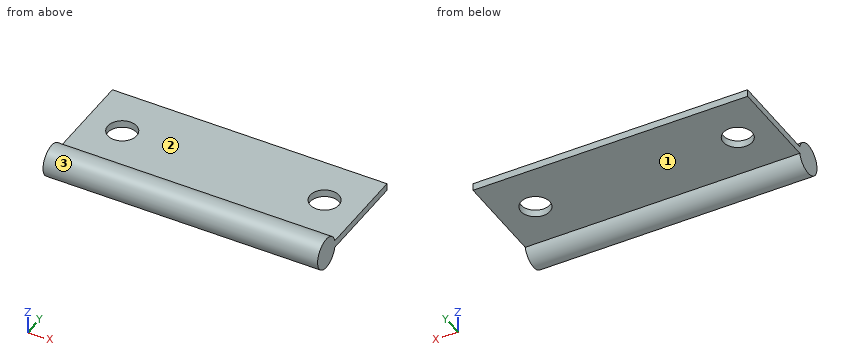
```python
from build123d import *

# Parameters (mm, degrees)
SKETCH_1_W          = 38
SKETCH_1_H          = 30
SKETCH_1_R          = 2
EXTRUDE_1_DEPTH     = 1
SKETCH_2_W          = 38
SKETCH_2_H          = 15
CUT_EXTRUDE_1_DEPTH = 1
SKETCH_4_R          = 2.15
EXTRUDE_2_DEPTH     = 38


with BuildPart() as part:
    # 草图1 → 凸台-拉伸1 (new body)
    with BuildSketch(Plane.XY):
        with Locations((-26.818488663, 4.019613274)):
            Rectangle(SKETCH_1_W, SKETCH_1_H)
        with Locations((-40.818488663, 12.519613274)):
            Circle(SKETCH_1_R, mode=Mode.SUBTRACT)
        with Locations((-12.818488663, 12.519613274)):
            Circle(SKETCH_1_R, mode=Mode.SUBTRACT)
        with Locations((-40.818488663, -4.480386726)):
            Circle(SKETCH_1_R, mode=Mode.SUBTRACT)
        with Locations((-12.818488663, -4.480386726)):
            Circle(SKETCH_1_R, mode=Mode.SUBTRACT)
    extrude(amount=EXTRUDE_1_DEPTH)

    # 草图2 → 切除-拉伸1 (cut)
    with BuildSketch(Plane.XY.offset(1)):
        with Locations((-26.818488663, -3.480386726)):
            Rectangle(SKETCH_2_W, SKETCH_2_H)
    extrude(amount=-CUT_EXTRUDE_1_DEPTH, mode=Mode.SUBTRACT)

    # 草图4 → 凸台-拉伸2 (add)
    with BuildSketch(Plane.ZY.offset(45.818488663)):
        with Locations((0.5, 4.019613274)):
            Circle(SKETCH_4_R)
    extrude(amount=-EXTRUDE_2_DEPTH)


solid = part.part
```
Here's how the part is built. I have some questions about the finished solid (model axes, mm). Face numbers are marked on the shaded views. A direction names the side the tool comes from. Coordinates: 2 decimals unless noted, no trailing zeros. Write each loop counter-clockwise with the first axis right and the second up, starting at its lowest first coordinate (ties: lowest second). Pieces come first, ordered by that corner, then holes. Notation, with made-up numbers: (-6.75, 16) - (14.25, 16) arc R27 cw to (14.25, 46) - close; hole circle Ø1 at (39.5, 3). An arc over 180 degrees is marked (long way). One line per item, written item: value.
1) Suppose I cut it at C-C on z = 0.5. Write out the boundary of the cut face in (x, y).
Model answer:
outline: (-45.82, 1.87) - (-7.82, 1.87) - (-7.82, 19.02) - (-45.82, 19.02) - close; hole circle Ø4 at (-40.82, 12.52); hole circle Ø4 at (-12.82, 12.52)
2) I'm going to push flat-ended pins straight in: P1, Ø4.5, axis at x = -40.82, y = 12.52, coming from the +Z side; P2, Ø4, axis at x = -29, y = 14, coming from the -Z side; P3, Ø1, axis at x = -31, z = -0.5, coming from the -Y side; P4, Ø3, axis at x = -12.82, y = 12.52, coming from the -Z side. Where does each tip first touch, or does it pass through?
Model answer:
P1: stops at z = 1
P2: stops at z = 0
P3: stops at y = 1.93
P4: passes through
3) Suppose I cut it at A-A on x = -13.5. Write out the boundary of the cut face in (y, z).
Model answer:
outline: (6.11, 0) - (10.64, 0) - (10.64, 1) - (6.11, 1) arc R2.15 ccw (long way) to start; (14.4, 0) - (19.02, 0) - (19.02, 1) - (14.4, 1) - close
4) Suppose I cut it at D-D on y = 13.75. Write out the boundary of the cut face in (x, z).
Model answer:
outline: (-45.82, 0) - (-42.4, 0) - (-42.4, 1) - (-45.82, 1) - close; (-39.24, 0) - (-14.4, 0) - (-14.4, 1) - (-39.24, 1) - close; (-11.24, 0) - (-7.82, 0) - (-7.82, 1) - (-11.24, 1) - close
5) On a 3-axis mill with a long thin cutter (end or side, diameter ignored), from which of +Z, -Z, +X, -X, +Y, -Y can I reach the whole of each face in a straight line? I mean the marked faces 1, 2 and 3. Say none if no direction works.
Model answer:
face 1: -Z, +X, -X, +Y
face 2: +Z, +X, -X, +Y
face 3: +X, -X
6) I need wall thicknesses on line 1 along X through (y, z) = (12.5, 0.6); line 2 along Z through (x, y) = (-41.5, 7); line 3 along Y through (x, z) = (-11.5, 0.15). Which ranges of each line are inside material? Lowest first, please.
Model answer:
line 1: x = -45.82 to -42.82, -38.82 to -14.82, -10.82 to -7.82
line 2: z = 0 to 1
line 3: y = 1.9 to 11.02, 14.02 to 19.02
7) Suppose I cut it at B-B on y = 11.25. Write out the boundary of the cut face in (x, z).
Model answer:
outline: (-45.82, 0) - (-42.36, 0) - (-42.36, 1) - (-45.82, 1) - close; (-39.27, 0) - (-14.36, 0) - (-14.36, 1) - (-39.27, 1) - close; (-11.27, 0) - (-7.82, 0) - (-7.82, 1) - (-11.27, 1) - close
